from build123d import *

# Parameters (mm, degrees)
F0_R     = 3.592825
F1_DEPTH = 3.175


with BuildPart() as f1:
    # F0 (on Top) → F1 (new body)
    with BuildSketch(Plane.XY):
        with BuildLine():
            ThreePointArc((0, 4.7625), (3.367596, 3.367596), (4.7625, 0))
            Line((4.7625, 0), (58.7375, 0))
            ThreePointArc((58.7375, 0), (60.132404, 3.367596), (63.5, 4.7625))
            Line((63.5, 4.7625), (63.5, 20.6375))
            ThreePointArc((63.5, 20.6375), (60.132404, 22.032404), (58.7375, 25.4))
            Line((58.7375, 25.4), (4.7625, 25.4))
            ThreePointArc((4.7625, 25.4), (3.367596, 22.032404), (0, 20.6375))
            Line((0, 20.6375), (0, 4.7625))
        make_face()
        with Locations((5.697345, 13.27287)):
            Circle(F0_R, mode=Mode.SUBTRACT)
    extrude(amount=F1_DEPTH)


solid = f1.part
Design review of the part built by this model. Coordinates are the model's own, in mm. Give positions to 0.01 mm unless a question says otherwise; leave off trailing zeros. Loops run counter-clockwise (first coordinate to the right, second up) from the corner with the lowest first, then second, coordinate; pieces in that order, holes last. Notation, with made-up numbers: (-9, -18) - (21, -18) arc R28 cw to (21, 5) - close; hole circle Ø9 at (46, 25). An arc over 180 degrees is marked (long way). Write item = value, one per line.
1) To check wall thickness, follow line 1 (X direction, y = 1.75, z = 1.5); line 2 (X direction, y = 1.5, z = 1.8); line 3 (X direction, y = 12.5, z = 0.9). State the ranges of each line that lie inside material, in increasing order.
Result sheet:
line_1 = 4.43 to 59.07
line_2 = 4.52 to 58.98
line_3 = 0 to 2.19, 9.21 to 63.5
2) Take a section at A-A on y = 11. State the section outline as (x, z) points (3 decimals).
Result sheet:
outline = (0, 0) - (2.915, 0) - (2.915, 3.175) - (0, 3.175) - close; (8.48, 0) - (63.5, 0) - (63.5, 3.175) - (8.48, 3.175) - close
3) Take a section at D-D on y = 22.5. State the section outline as (x, z) points (3 decimals).
Result sheet:
outline = (3.778, 0) - (59.722, 0) - (59.722, 3.175) - (3.778, 3.175) - close
4) Take a section at C-C on z = 2.15. State the section outline as (x, y) points (1 decimal).
Result sheet:
outline = (0, 4.8) arc R4.8 cw to (4.8, 0) - (58.7, 0) arc R4.8 cw to (63.5, 4.8) - (63.5, 20.6) arc R4.8 cw to (58.7, 25.4) - (4.8, 25.4) arc R4.8 cw to (0, 20.6) - close; hole circle Ø7.2 at (5.7, 13.3)
5) Take a section at B-B on x = 5.5. State the section outline as (y, z) points (3 decimals), and give its area (3 significant figures).
Result sheet:
outline = (0, 0) - (9.685, 0) - (9.685, 3.175) - (0, 3.175) - close; (16.86, 0) - (25.4, 0) - (25.4, 3.175) - (16.86, 3.175) - close
area = 57.9 mm2
6) Draft analysis for pull direction X (two halves, no side actions). For faces 1 (the face through (3.33, 3.404, 1.565)), 2 (the face through (60.17, 21.996, 1.565)), 3 (the face through (2.846, 11.087, 1.565)), state which applies: +X half, -X half, draft (parallel to the pull), parting line (faces both ways), or undercut.
Result sheet:
face_1 = -X half
face_2 = +X half
face_3 = undercut
